Design review of the part built by this model. Coordinates are the model's own, in mm. A direction names the side the tool comes from. Give positions to 0.01 mm unless a question says otherwise; leave off trailing zeros. Loops run counter-clockwise (first coordinate to the right, second up) from the corner with the lowest first, then second, coordinate; pieces in that order, holes last. Notation, with made-up numbers: (56, -32) -> (69, -32) arc R22 cw to (69, -22) -> close; hole circle Ø7 at (14, 12.5). An arc over 180 degrees is marked (long way). Answer in a Markdown table with one row per item. Add a question column.
(1) Consider section B-B on y = 0. Write out the cut boundary in (x, z).
(2) Draft analysis for pull direction X (two halves, no side actions). For faces 1 (the flat face through (17, 0, 0)), 2 (the flat face through (4, -6.5, -5.6)), 3 (the flat face through (1, 17.175, -8)), state which applies: +X half, -X half, draft (parallel to the pull), parting line (faces both ways), or undercut.
(3) Consider section C-C on x = 9. Write out the cut boundary in (y, z), then the cut area to 3 significant figures.
(4) For pin 1 (8 mm diameter, centred on x = 15, z = -6.5, fed in from -Y); pin 2 (3 mm diameter, centred on x = 1.5, z = 7.5, fed in from +Y); pin 3 (0.8 mm diameter, centred on y = 6.5, z = -7.5, fed in from -X), all flat-tipped, find the tip position at first contact; note any pin that passes through.
(5) For line 1 (Z direction, x = 4.5, y = 0.5); line 2 (X direction, y = 2, z = 3.25); line 3 (X direction, y = 2, z = -7.5), list the stretches that pass through material, from the lowest coordinate up.
(6) Consider section A-A on z = 0. Write out the cut boundary in (x, y), then the cut area to 3 significant figures.
(7) Consider section D-D on y = -14.5. Write out the cut boundary in (x, z).
(8) For faces 4 (the cylindrical face through (6, 22, 0)), 5 (the flat face through (2.71, -13.31, 3.7)), 6 (the flat face through (5, -6.943, 6)), list the 3-axis set-ups (+Z, -Z, +X, -X, +Y, -Y) from which the entire face can be reached by the end or side of a thin tool; tool diameter is ignored.
from build123d import *

# Parameters (mm, degrees)
SKETCH1_R           = 22
BOSS_EXTRUDE1_DEPTH = 12
CUT_EXTRUDE2_DEPTH  = 5.5
SKETCH15_W          = 18
SKETCH15_H          = 24.118038922
CUT_EXTRUDE3_DEPTH  = 3
SKETCH16_R          = 8.55
BOSS_EXTRUDE2_DEPTH = 5
SKETCH17_W          = 4
SKETCH17_H          = 1.75
BOSS_EXTRUDE3_DEPTH = 1
SKETCH18_W          = 4.25
SKETCH18_H          = 1.737607108
BOSS_EXTRUDE4_DEPTH = 1
CUT_EXTRUDE4_DEPTH  = 12


# Read off the part's stored shape, not the designer's step: Cut-Extrude4
with BuildPart() as part:
    # Sketch1 → Boss-Extrude1 (new body)
    with BuildSketch(Plane(origin=(0, 0, 0), x_dir=(0, 0, -1), z_dir=(1, 0, 0))):
        Circle(SKETCH1_R)
    extrude(amount=BOSS_EXTRUDE1_DEPTH)

    # Sketch13 → Cut-Extrude2 (cut)
    with BuildSketch(Plane(origin=(0, 0, 0), x_dir=(0, 0, -1), z_dir=(1, 0, 0))):
        with BuildLine():
            Line((-2.670420152, -16.85816067), (-2.670420152, -16.530371213))
            Line((-2.670420152, -16.530371213), (-4.762392892, -10))
            Line((-4.762392892, -10), (-4.762392892, -6.943148259))
            Line((-4.762392892, -6.943148259), (-6.5, -6.943148259))
            Line((-6.5, -6.943148259), (-6.5, 19.556851741))
            Line((-6.5, 19.556851741), (6.5, 19.556851741))
            Line((6.5, 19.556851741), (6.5, -6.943148259))
            Line((6.5, -6.943148259), (4.762392892, -6.943148259))
            Line((4.762392892, -6.943148259), (4.762392892, -10))
            Line((4.762392892, -10), (2.670420152, -16.530371213))
            Line((2.670420152, -16.530371213), (2.670420152, -16.85816067))
            Line((2.670420152, -16.85816067), (2.670420152, -21.837327131))
            ThreePointArc((2.670420152, -21.837327131), (1.836835043, -21.92318492), (1.000584871, -21.977234355))
            Line((1.000584871, -21.977234355), (0, -25.25))
            Line((0, -25.25), (-1.000584871, -21.977234355))
            ThreePointArc((-1.000584871, -21.977234355), (-1.836835043, -21.92318492), (-2.670420152, -21.837327131))
            Line((-2.670420152, -21.837327131), (-2.670420152, -16.85816067))
        make_face()
    extrude(amount=CUT_EXTRUDE2_DEPTH, mode=Mode.SUBTRACT)

    # Sketch15 → Cut-Extrude3 (cut)
    with BuildSketch(Plane.ZY):
        with Locations((0, 5.115871202)):
            Rectangle(SKETCH15_W, SKETCH15_H)
    extrude(amount=-CUT_EXTRUDE3_DEPTH, mode=Mode.SUBTRACT)

    # Sketch16 → Boss-Extrude2 (add)
    with BuildSketch(Plane(origin=(12, 0, 0), x_dir=(0, 0, -1), z_dir=(1, 0, 0))):
        Circle(SKETCH16_R)
    extrude(amount=BOSS_EXTRUDE2_DEPTH)

    # Sketch17 → Boss-Extrude3 (add)
    with BuildSketch(Plane(origin=(0, -6.943148259, 0), x_dir=(1, 0, 0), z_dir=(0, 1, 0))):
        with Locations((2, 5.637392892)):
            Rectangle(SKETCH17_W, SKETCH17_H)
    extrude(amount=BOSS_EXTRUDE3_DEPTH)

    # Sketch18 → Boss-Extrude4 (add)
    with BuildSketch(Plane(origin=(0, -6.943148259, 0), x_dir=(1, 0, 0), z_dir=(0, 1, 0))):
        with Locations((2.125, -5.631196446)):
            Rectangle(SKETCH18_W, SKETCH18_H)
    extrude(amount=BOSS_EXTRUDE4_DEPTH)

    # Cut-Extrude4 outline → Cut-Extrude4 (cut)
    with BuildSketch(Plane(origin=(0, 0, 0), x_dir=(0, 0, -1), z_dir=(1, 0, 0))):
        with BuildLine():
            ThreePointArc((11, -19.052558883), (22, 0), (11, 19.052558883))
            Line((11, 19.052558883), (11, -19.052558883))
        make_face()
        with BuildLine():
            Line((-11, -19.052558883), (-11, 19.052558883))
            ThreePointArc((-11, 19.052558883), (-22, 0), (-11, -19.052558883))
        make_face()
    extrude(amount=CUT_EXTRUDE4_DEPTH, mode=Mode.SUBTRACT)


solid = part.part
Values follow:
| question | item | result |
|---|---|---|
| 1 | outline | (0, -11) -> (12, -11) -> (12, -8.55) -> (17, -8.55) -> (17, 8.55) -> (12, 8.55) -> (12, 11) -> (0, 11) -> (0, 9) -> (3, 9) -> (3, 6.5) -> (5.5, 6.5) -> (5.5, -6.5) -> (3, -6.5) -> (3, -9) -> (0, -9) -> close |
| 2 | face 1 | +X half |
| 2 | face 2 | undercut |
| 2 | face 3 | draft |
| 3 | outline | (-19.05, -11) -> (19.05, -11) arc R22 ccw to (19.05, 11) -> (-19.05, 11) arc R22 ccw to start |
| 3 | area | 926 mm2 |
| 4 | pin 1 | y = -21.66 |
| 4 | pin 2 | y = 21.17 |
| 4 | pin 3 | x = 3 |
| 5 | line 1 | -11 to -6.5, 6.5 to 11 |
| 5 | line 2 | 5.5 to 17 |
| 5 | line 3 | 3 to 17 |
| 6 | outline | (0, 19.56) -> (5.5, 19.56) -> (5.5, -22) -> (12, -22) -> (12, -8.55) -> (17, -8.55) -> (17, 8.55) -> (12, 8.55) -> (12, 22) -> (0, 22) -> close |
| 6 | area | 385 mm2 |
| 7 | outline | (0, -11) -> (12, -11) -> (12, 11) -> (0, 11) -> (0, 3.32) -> (5.5, 3.32) -> (5.5, -3.32) -> (0, -3.32) -> close |
| 8 | face 4 | +X, -X, +Y |
| 8 | face 5 | -X |
| 8 | face 6 | none |
